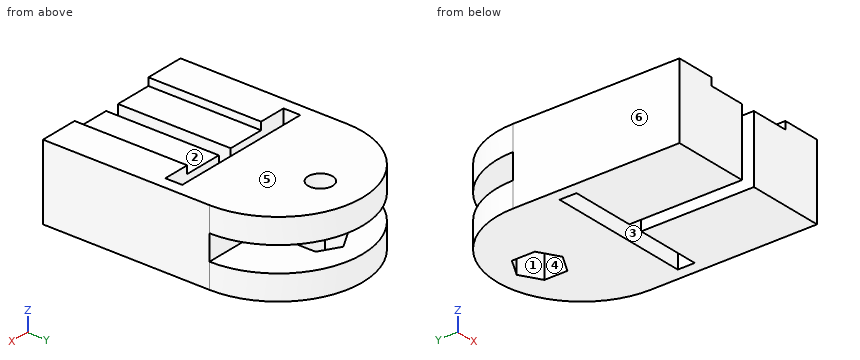
from build123d import *

# Parameters (mm, degrees)
F0_R      = 1.6
F1_DEPTH  = 9.78
F2_W      = 11.0329598772
F2_H      = 3.28
F3_DEPTH  = 22
F4_W      = 5.05
F4_H      = 15.2
F4_W_2    = 4.86
F5_DEPTH  = 1
F6_R      = 1.6
F7_DEPTH  = 3.26
F9_R      = 1.6
F10_DEPTH = 3.26
F11_DEPTH = 0.5


with BuildPart() as f1:
    # F0 (on Top) → F1 (new body)
    with BuildSketch(Plane.XY):
        with BuildLine():
            Line((-33.4101816105, 245.5555587423), (-33.4101816105, 223.8355587423))
            Line((-33.4101816105, 223.8355587423), (-23.4101816105, 223.8355587423))
            Line((-23.4101816105, 223.8355587423), (-23.4101816105, 239.0355587423))
            Line((-23.4101816105, 239.0355587423), (-31.8601816105, 239.0355587423))
            Line((-31.8601816105, 239.0355587423), (-31.8601816105, 240.7355587423))
            Line((-31.8601816105, 240.7355587423), (-23.4101816105, 240.7355587423))
            Line((-23.4101816105, 240.7355587423), (-21.5101816105, 240.7355587423))
            Line((-21.5101816105, 240.7355587423), (-12.9601816105, 240.7355587423))
            Line((-12.9601816105, 240.7355587423), (-12.9601816105, 239.0355587423))
            Line((-12.9601816105, 239.0355587423), (-21.5101816105, 239.0355587423))
            Line((-21.5101816105, 239.0355587423), (-21.5101816105, 223.8355587423))
            Line((-21.5101816105, 223.8355587423), (-11.4101816105, 223.8355587423))
            Line((-11.4101816105, 223.8355587423), (-11.4101816105, 245.5555587423))
            ThreePointArc((-11.4101816105, 245.5555587423), (-22.4101816105, 256.5555587423), (-33.4101816105, 245.5555587423))
        make_face()
        with Locations((-22.4101816105, 251.0555587423)):
            Circle(F0_R, mode=Mode.SUBTRACT)
    extrude(amount=F1_DEPTH)

    # F2 (on face) → F3 (cut)
    with BuildSketch(Plane(origin=(-33.4101816105, 0, 0), x_dir=(0, -1, 0), z_dir=(-1, 0, 0))):
        with Locations((-251.0720386809, 4.89)):
            Rectangle(F2_W, F2_H)
    extrude(amount=-F3_DEPTH, mode=Mode.SUBTRACT)

    # F4 (on face) → F5 (cut)
    with BuildSketch(Plane.XY.offset(9.78)):
        with Locations((-18.9851816105, 231.4355587423)):
            Rectangle(F4_W, F4_H)
        with Locations((-25.8401816105, 231.4355587423)):
            Rectangle(F4_W_2, F4_H)
    extrude(amount=-F5_DEPTH, mode=Mode.SUBTRACT)

    # F9 (on face) → F10 (cut)
    with BuildSketch(Plane(origin=(0, 0, 0), x_dir=(1, 0, 0), z_dir=(0, 0, -1))):
        Polygon((-22.4101816105, -254.0555587423), (-19.8121053991, -252.5555587423), (-19.8121053991, -249.5555587423), (-22.4101816105, -248.0555587423), (-25.0082578218, -249.5555587423), (-25.0082578218, -252.5555587423), align=None)
        with Locations((-22.4101816105, -251.0555587423)):
            Circle(F9_R, mode=Mode.SUBTRACT)
    extrude(amount=-F10_DEPTH, mode=Mode.SUBTRACT)

    # F11 (cut): faces of the model
    f11_faces = [f1.faces().sort_by_distance(p)[0] for p in [
        (-27.7473388211, 239.0355587423, 4.6156990782),
        (-17.1227008611, 239.0355587423, 4.6078340058),
    ]]
    extrude(f11_faces, amount=-F11_DEPTH, mode=Mode.SUBTRACT)


with BuildPart() as f7:
    # F6 (on face) → F7 (new body)
    with BuildSketch(Plane.XY.offset(3.25)):
        with BuildLine():
            Line((-11.4101816105, 334.1924881189), (-33.4101816105, 334.1924881189))
            Line((-33.4101816105, 334.1924881189), (-33.4101816105, 290.1924881189))
            ThreePointArc((-33.4101816105, 290.1924881189), (-22.4101816105, 279.1924881189), (-11.4101816105, 290.1924881189))
            Line((-11.4101816105, 290.1924881189), (-11.4101816105, 334.1924881189))
        make_face()
        with Locations((-22.4101816105, 284.5924881189)):
            Circle(F6_R, mode=Mode.SUBTRACT)
    extrude(amount=F7_DEPTH)


solid = f1.part
Geometry check sheet. Reference: the model listing, model coordinates, mm. Face numbers are marked on the shaded views. A direction names the side the tool comes from. Coordinates: 2 decimals unless noted, no trailing zeros. Order: outer loops, then holes, each group sorted by start corner. A loop starts at its lowest first (then second) coordinate and runs counter-clockwise, first axis right, second up. Notation, with made-up numbers: M -36.75,39 L 8.25,39 A22 ccw 8.25,56 Z; hole C -14.75,33 d3. An arc over 180 degrees is marked long. Use CSV: the item, a comma, the result in double quotes.
Item 1: Tool access check on the marked faces 1, 2 and 3. Record the directions out of +Z, -Z, +X, -X, +Y, -Y that give a thin tool (end or side, any length) a straight path to the whole face; none if there is none.
Returned:
face 1,"-Z"
face 2,"+Z, -Y"
face 3,"+Z, -Z"
Item 2: Cross-section at B-B on x = -30. Record the cut outline in (y, z).
Returned:
outline,"M 223.84,0 L 238.54,0 L 238.54,9.78 L 223.84,9.78 Z; M 240.74,0 L 253.52,0 L 253.52,3.25 L 245.56,3.25 L 245.56,6.53 L 253.52,6.53 L 253.52,9.78 L 240.74,9.78 Z"
Item 3: Thickness scan on line 1 along Y through (x, z) = (-30, 4); line 2 along X through (y, z) = (235, 1.5); line 3 along Z through (x, y) = (-18, 249). Record the ranges inside material, lowest first.
Returned:
line 1,"y = 223.84 to 238.54, 240.74 to 245.56"
line 2,"x = -33.41 to -23.41, -21.51 to -11.41"
line 3,"z = 0 to 3.25, 6.53 to 9.78"
Item 4: Cross-section at A-A on y = 227. Record the cut outline in (x, z).
Returned:
outline,"M -33.41,0 L -23.41,0 L -23.41,8.78 L -28.27,8.78 L -28.27,9.78 L -33.41,9.78 Z; M -21.51,0 L -11.41,0 L -11.41,9.78 L -16.46,9.78 L -16.46,8.78 L -21.51,8.78 Z"
Item 5: Mould release check, pull along X, two halves, no side actions. Record for the marked faces 4, 5 and 6: pulls with the +X half, pulls with the -X half, needs draft (parallel to the pull), parting line crosses it, or undercut.
Returned:
face 4,"undercut"
face 5,"needs draft"
face 6,"pulls with the -X half"
Item 6: Cross-section at C-C on z = 4.5. Record the cut outline in (x, y), then the cut area to 3 significant figures.
Returned:
outline,"M -33.41,223.84 L -23.41,223.84 L -23.41,238.54 L -31.86,238.54 L -31.86,240.74 L -12.96,240.74 L -12.96,238.54 L -21.51,238.54 L -21.51,223.84 L -11.41,223.84 L -11.41,245.56 L -33.41,245.56 Z"
area,"408 mm2"
Item 7: Gauge pin test, flat ends, axial feed: pin 1 Ø4 at (x, z) = (-28, 5.5) entering from +Y; pin 2 Ø1 at (x, z) = (-27.5, 3.5) entering from +Y; pin 3 Ø1 at (y, z) = (248, 6) entering from +X; pin 4 Ø3.5 at (y, z) = (251.5, 1) entering from +X. Record the tip position at first contact, or that the pin passes through.
Returned:
pin 1,"stops at y = 255.85"
pin 2,"stops at y = 255.52"
pin 3,"passes through"
pin 4,"stops at x = -12.24"
Item 8: Cross-section at D-D on y = 252. Record the cut outline in (x, z).
Returned:
outline,"M -31.32,0 L -25.01,0 L -25.01,3.25 L -31.32,3.25 Z; M -31.32,6.53 L -23.7,6.53 L -23.7,9.78 L -31.32,9.78 Z; M -21.12,6.53 L -13.5,6.53 L -13.5,9.78 L -21.12,9.78 Z; M -19.81,0 L -13.5,0 L -13.5,3.25 L -19.81,3.25 Z"
